Build history of the part. All positions in model axes, mm. A direction names the side the tool comes from. Round coordinates to 2 decimals unless told otherwise and drop trailing zeros. Write each loop counter-clockwise with the first axis right and the second up, starting at its lowest first coordinate (ties: lowest second). Pieces come first, ordered by that corner, then holes. Notation, with made-up numbers: (27, 19.5) - (48, 19.5) arc R9 ccw to (48, 25.5) - close; hole circle Ø6 at (23.5, 89.25). An arc over 180 degrees is marked (long way). One line per question, with ' | ' between items.
from build123d import *

# Parameters (mm, degrees)
F2_R = 1.25
F3_R = 0.3


with BuildPart() as f1:
    # F0 (on Front) → F1 (revolve)
    with BuildSketch(Plane.XZ):
        Polygon((0, -22.6), (0, -23), (2, -23), (3.4, -17), (3.4, -12), (5.4, -12), (5.4, -11), (3.4, -11), (3.4, 0), (3, 0), (3, -16.953952), (1.682589, -22.6), align=None)
    revolve(axis=Axis((0, 0, -11.5), (0, 0, -1)))

    # F2
    f2_edges = [f1.edges().sort_by_distance(p)[0] for p in [
        (-2, 0, -23),
        (-3.4, 0, -17),
    ]]
    fillet(f2_edges, radius=F2_R)

    # F3
    f3_edges = [f1.edges().sort_by_distance(p)[0] for p in [
        (-5.4, 0, -11),
        (-5.4, 0, -12),
    ]]
    fillet(f3_edges, radius=F3_R)


solid = f1.part
Q1. Which spindle directions (+Z, -Z, +X, -X, +Y, -Y) get a long thin tool onto all of the face, cutting with end or side? Do faces 5 (the cylindrical face through (-2.698, 2.069, -14.394)), 6 (the flat face through (1, 3, 0)), 7 (the cylindrical face through (-3, 0, -9)). Say none if no direction does.
Found:
face 5: -Z | face 6: +Z, +X, -X, +Y, -Y | face 7: +Z
Q2. Pull direction Y, two halves, no side cores. Call faces 1 (the flat face through (0, 0, -22.6)), 2 (the conical face through (1.18, -1.84, -20.44)), 3 (the cylindrical face through (-0.74, 3.32, -5.42)), 4 (the flat face through (0, 0, -23)): +Y half, -Y half, draft (parallel to the pull), parting line (faces both ways), or undercut.
Found:
face 1: undercut | face 2: undercut | face 3: parting line | face 4: draft
Q3. Drop flat-ended pins along their axis: pin 1 (1.7 mm diameter, centred on x = -0.5, y = 0, fed in from +Z); pin 2 (4 mm diameter, centred on x = 3.5, y = 0.5, fed in from -Z); pin 3 (1.5 mm diameter, centred on x = -3.5, z = -4, fed in from +Y). Give the stop position or say it passes through.
Found:
pin 1: z = -22.6 | pin 2: z = -22.88 | pin 3: y = 2
Q4. Drill centre lines: L1, parallel to X at y = 0, z = -5; L2, parallel to Z at x = 0.5, y = -4.5. Where is each one in solid material? Low to high. Write a range as from..to.
Found:
L1: -3.4..-3, 3..3.4 | L2: -12..-11
Q5. Saw through at A-A, the plane z = -14.5. List the corners of the cut face in (x, y), then the cut area to 3 significant figures.
Found:
outline: circle Ø6.8 at (0, 0); hole circle Ø6 at (0, 0) | area: 8.04 mm^2
